Can you work these out from the model? Positions are in its coordinate system, mm. Give positions to 0.01 mm unless a question says otherwise; leave off trailing zeros. Order: outer loops, then holes, each group sorted by start corner. A loop starts at its lowest first (then second) coordinate and runs counter-clockwise, first axis right, second up. Notation, with made-up numbers: M 27.5,77 L 32.5,77 A28 cw 32.5,100 Z; hole C -2,50 d10. An arc over 180 degrees is marked long. Answer as a JSON object with one key per item and string values.
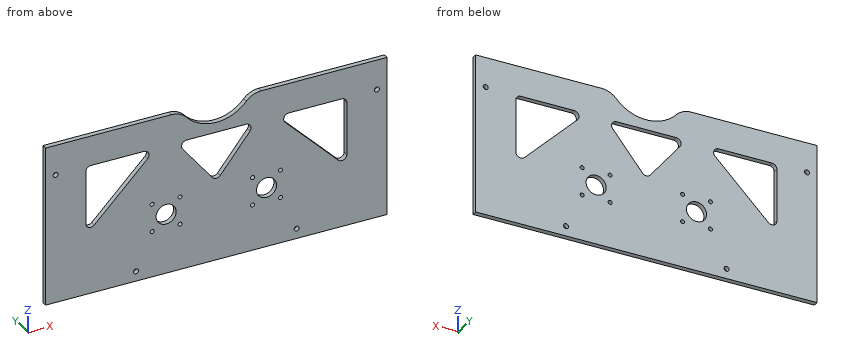
```python
from build123d import *

# Parameters (mm, degrees)
BOSS_EXTRUDE1_DEPTH = 3.175
SKETCH2_R           = 6.35
CUT_EXTRUDE1_DEPTH  = 315.453256661
FILLET1_R           = 12.7
SKETCH3_R           = 1.27
CUT_EXTRUDE2_DEPTH  = 315.453256661
SKETCH4_R           = 1.5875
CUT_EXTRUDE3_DEPTH  = 315.453256661
CUT_EXTRUDE4_DEPTH  = 315.453256661
CUT_EXTRUDE5_DEPTH  = 315.453256661
FILLET2_R           = 3.175


with BuildPart() as part:
    # Sketch1 → Boss-Extrude1 (new body)
    with BuildSketch(Plane(origin=(0, 0, 0), x_dir=(1, 0, 0), z_dir=(0, 1, 0))):
        with BuildLine():
            Line((0, 228.6), (0, 127))
            Line((0, 127), (85.952954744, 127))
            ThreePointArc((85.952954744, 127), (107.95, 139.7), (129.947045256, 127))
            Line((129.947045256, 127), (215.9, 127))
            Line((215.9, 127), (215.9, 228.6))
            Line((215.9, 228.6), (0, 228.6))
        make_face()
    extrude(amount=BOSS_EXTRUDE1_DEPTH)

    # Sketch2 → Cut-Extrude1 (cut, through all)
    with BuildSketch(Plane(origin=(0, 3.175, 0), x_dir=(1, 0, 0), z_dir=(0, 1, 0))):
        with Locations(Location((76.2, 190.5, 0), (0, 0, 270))):
            Circle(SKETCH2_R)
        with Locations(Location((139.7, 190.5, 0), (0, 0, 270))):
            Circle(SKETCH2_R)
    extrude(amount=-CUT_EXTRUDE1_DEPTH, mode=Mode.SUBTRACT)

    # Fillet1
    fillet1_edges = [part.edges().sort_by_distance(p)[0] for p in [
        (85.952954744, 1.5875, -127),
        (129.947045256, 1.5875, -127),
    ]]
    fillet(fillet1_edges, radius=FILLET1_R)

    # Sketch3 → Cut-Extrude2 (cut, through all)
    with BuildSketch(Plane(origin=(0, 3.175, 0), x_dir=(1, 0, 0), z_dir=(0, 1, 0))):
        with Locations(Location((85.038834765, 199.338834765, 0), (0, 0, 270))):
            Circle(SKETCH3_R)
        with Locations(Location((67.361165235, 181.661165235, 0), (0, 0, 270))):
            Circle(SKETCH3_R)
        with Locations(Location((67.361165235, 199.338834765, 0), (0, 0, 270))):
            Circle(SKETCH3_R)
        with Locations(Location((85.038834765, 181.661165235, 0), (0, 0, 270))):
            Circle(SKETCH3_R)
        with Locations(Location((130.861165235, 181.661165235, 0), (0, 0, 270))):
            Circle(SKETCH3_R)
        with Locations(Location((148.538834765, 181.661165235, 0), (0, 0, 270))):
            Circle(SKETCH3_R)
        with Locations(Location((148.538834765, 199.338834765, 0), (0, 0, 270))):
            Circle(SKETCH3_R)
        with Locations(Location((130.861165235, 199.338834765, 0), (0, 0, 270))):
            Circle(SKETCH3_R)
    extrude(amount=-CUT_EXTRUDE2_DEPTH, mode=Mode.SUBTRACT)

    # Sketch4 → Cut-Extrude3 (cut, through all)
    with BuildSketch(Plane(origin=(0, 3.175, 0), x_dir=(1, 0, 0), z_dir=(0, 1, 0))):
        with Locations(Location((6.35, 146.05, 0), (0, 0, 270))):
            Circle(SKETCH4_R)
        with Locations(Location((57.15, 222.25, 0), (0, 0, 270))):
            Circle(SKETCH4_R)
        with Locations(Location((158.75, 222.25, 0), (0, 0, 270))):
            Circle(SKETCH4_R)
        with Locations(Location((209.55, 146.05, 0), (0, 0, 270))):
            Circle(SKETCH4_R)
    extrude(amount=-CUT_EXTRUDE3_DEPTH, mode=Mode.SUBTRACT)

    # Sketch5 → Cut-Extrude4 (cut, through all)
    with BuildSketch(Plane(origin=(0, 3.175, 0), x_dir=(1, 0, 0), z_dir=(0, 1, 0))):
        Polygon((25.4, 190.5), (25.4, 146.05), (69.85, 146.05), align=None)
        Polygon((190.5, 146.05), (146.05, 146.05), (190.5, 190.5), align=None)
    extrude(amount=-CUT_EXTRUDE4_DEPTH, mode=Mode.SUBTRACT)

    # Sketch6 → Cut-Extrude5 (cut, through all)
    with BuildSketch(Plane(origin=(0, 3.175, 0), x_dir=(1, 0, 0), z_dir=(0, 1, 0))):
        Polygon((82.55, 146.05), (133.35, 146.05), (107.95, 177.8), align=None)
    extrude(amount=-CUT_EXTRUDE5_DEPTH, mode=Mode.SUBTRACT)

    # Fillet2
    fillet2_edges = [part.edges().sort_by_distance(p)[0] for p in [
        (25.4, 1.5875, -190.5),
        (69.85, 1.5875, -146.05),
        (25.4, 1.5875, -146.05),
        (190.5, 1.5875, -190.5),
        (190.5, 1.5875, -146.05),
        (146.05, 1.5875, -146.05),
        (82.55, 1.5875, -146.05),
        (107.95, 1.5875, -177.8),
        (133.35, 1.5875, -146.05),
    ]]
    fillet(fillet2_edges, radius=FILLET2_R)


solid = part.part
```
1) I want a section at C-C on z = -134. Write out the boundary of the cut face in (x, y) (3 decimals), and give its area (3 significant figures).
Results found:
{"outline": "M 0,0 L 91.917,0 L 91.917,3.175 L 0,3.175 Z; M 123.983,0 L 215.9,0 L 215.9,3.175 L 123.983,3.175 Z", "area": "584 mm²"}
2) I want a section at A-A on z = -169. Write out the boundary of the cut face in (x, y) (3 decimals), and give its area (3 significant figures).
Results found:
{"outline": "M 0,0 L 25.4,0 L 25.4,3.175 L 0,3.175 Z; M 46.9,0 L 100.91,0 L 100.91,3.175 L 46.9,3.175 Z; M 114.99,0 L 169,0 L 169,3.175 L 114.99,3.175 Z; M 190.5,0 L 215.9,0 L 215.9,3.175 L 190.5,3.175 Z", "area": "504 mm²"}
3) I want a section at D-D on z = -191. Write out the boundary of the cut face in (x, y) (3 decimals).
Results found:
{"outline": "M 0,0 L 69.87,0 L 69.87,3.175 L 0,3.175 Z; M 82.53,0 L 133.37,0 L 133.37,3.175 L 82.53,3.175 Z; M 146.03,0 L 215.9,0 L 215.9,3.175 L 146.03,3.175 Z"}
4) I need wall thicknesses on L1, parallel to X at y = 0.45, z = -190.5; L2, parallel to X at y = 2, z = -222.25; L3, parallel to Z at x = 85.5, y = 2.6. Which ranges of each line are inside material? Lowest first, please.
Results found:
{"L1": "x = 0 to 69.85, 82.55 to 133.35, 146.05 to 215.9", "L2": "x = 0 to 55.56, 58.74 to 157.16, 160.34 to 215.9", "L3": "z = -228.6 to -200.52, -198.16 to -182.84, -180.48 to -128.48"}
5) I'm going to push a flat-ended pin straight in: pin 1 Ø1 at (x, y) = (81, 1.5) entering from +Z. Where does the tip first touch, or does it pass through?
Results found:
{"pin 1": "stops at z = -127.04"}
6) I want a section at B-B on x = 139.7. Write out the boundary of the cut face in (y, z) (3 decimals), and give its area (3 significant figures).
Results found:
{"outline": "M 0,-228.6 L 3.175,-228.6 L 3.175,-196.85 L 0,-196.85 Z; M 0,-184.15 L 3.175,-184.15 L 3.175,-127 L 0,-127 Z", "area": "282 mm²"}
